Part model, mm, in its own coordinate system. A direction names the side the tool comes from. Coordinates: 2 decimals unless noted, no trailing zeros. Write each loop counter-clockwise with the first axis right and the second up, starting at its lowest first coordinate (ties: lowest second). Pieces come first, ordered by that corner, then holes. Notation, with made-up numbers: (8.5, 84.25) -> (57.5, 84.25) arc R18 cw to (57.5, 113.25) -> close; hole circle Ø8 at (89, -5). An arc over 180 degrees is marked (long way). Write item = value, one per line.
from build123d import *

# Parameters (mm, degrees)
SALIENTE_EXTRUIR1_DEPTH = 2
CORTAR_EXTRUIR1_START   = -2
CORTAR_EXTRUIR1_DEPTH   = 2


with BuildPart() as part:
    # Croquis1 → Saliente-Extruir1 (new body)
    with BuildSketch(Plane.XY):
        with BuildLine():
            Line((-39.554396855, 20.88242961), (-39.554396855, 1.28242961))
            ThreePointArc((-39.554396855, 1.28242961), (-38.763585164, -0.626758699), (-36.854396855, -1.41757039))
            Line((-36.854396855, -1.41757039), (-12.254396855, -1.41757039))
            ThreePointArc((-12.254396855, -1.41757039), (-10.345208546, -0.626758699), (-9.554396855, 1.28242961))
            Line((-9.554396855, 1.28242961), (-9.554396855, 20.88242961))
            ThreePointArc((-9.554396855, 20.88242961), (-10.345208546, 22.791617919), (-12.254396855, 23.58242961))
            Line((-12.254396855, 23.58242961), (-36.854396855, 23.58242961))
            ThreePointArc((-36.854396855, 23.58242961), (-38.763585164, 22.791617919), (-39.554396855, 20.88242961))
        make_face()
        with BuildLine():
            Line((-14.554396855, 18.90242961), (-34.554396855, 18.90242961))
            ThreePointArc((-34.554396855, 18.90242961), (-35.654396855, 17.80242961), (-34.554396855, 16.70242961))
            Line((-34.554396855, 16.70242961), (-14.554396855, 16.70242961))
            ThreePointArc((-14.554396855, 16.70242961), (-13.454396855, 17.80242961), (-14.554396855, 18.90242961))
        make_face(mode=Mode.SUBTRACT)
        with BuildLine():
            Line((-34.554396855, 3.26242961), (-14.554396855, 3.26242961))
            ThreePointArc((-14.554396855, 3.26242961), (-13.454396855, 4.36242961), (-14.554396855, 5.46242961))
            Line((-14.554396855, 5.46242961), (-34.554396855, 5.46242961))
            ThreePointArc((-34.554396855, 5.46242961), (-35.654396855, 4.36242961), (-34.554396855, 3.26242961))
        make_face(mode=Mode.SUBTRACT)
    extrude(amount=SALIENTE_EXTRUIR1_DEPTH)

    # Croquis2 → Cortar-Extruir1 (cut)
    with BuildSketch(Plane.XY.offset(2).offset(CORTAR_EXTRUIR1_START)):
        with BuildLine():
            Line((-39.554396855, 20.88242961), (-39.554396855, 1.28242961))
            ThreePointArc((-39.554396855, 1.28242961), (-38.763585164, -0.626758699), (-36.854396855, -1.41757039))
            Line((-36.854396855, -1.41757039), (-12.254396855, -1.41757039))
            ThreePointArc((-12.254396855, -1.41757039), (-10.345208546, -0.626758699), (-9.554396855, 1.28242961))
            Line((-9.554396855, 1.28242961), (-9.554396855, 20.88242961))
            ThreePointArc((-9.554396855, 20.88242961), (-10.345208546, 22.791617919), (-12.254396855, 23.58242961))
            Line((-12.254396855, 23.58242961), (-36.854396855, 23.58242961))
            ThreePointArc((-36.854396855, 23.58242961), (-38.763585164, 22.791617919), (-39.554396855, 20.88242961))
        make_face()
        with BuildLine():
            Line((-39.204396855, 20.88242961), (-39.204396855, 1.28242961))
            ThreePointArc((-39.204396855, 1.28242961), (-38.516097791, -0.379271326), (-36.854396855, -1.06757039))
            Line((-36.854396855, -1.06757039), (-12.254396855, -1.06757039))
            ThreePointArc((-12.254396855, -1.06757039), (-10.592695919, -0.379271326), (-9.904396855, 1.28242961))
            Line((-9.904396855, 1.28242961), (-9.904396855, 20.88242961))
            ThreePointArc((-9.904396855, 20.88242961), (-10.592695919, 22.544130546), (-12.254396855, 23.23242961))
            Line((-12.254396855, 23.23242961), (-36.854396855, 23.23242961))
            ThreePointArc((-36.854396855, 23.23242961), (-38.516097791, 22.544130546), (-39.204396855, 20.88242961))
        make_face(mode=Mode.SUBTRACT)
    extrude(amount=CORTAR_EXTRUIR1_DEPTH, mode=Mode.SUBTRACT)


solid = part.part
Q1. Saw through at C-C on y = 18.5. Give the cut face in (x, z), and give its area (3 significant figures).
Model answer:
outline = (-39.2, 0) -> (-35.4, 0) -> (-35.4, 2) -> (-39.2, 2) -> close; (-13.7, 0) -> (-9.9, 0) -> (-9.9, 2) -> (-13.7, 2) -> close
area = 15.2 mm²
Q2. Which spindle directions (+Z, -Z, +X, -X, +Y, -Y) get a long thin tool onto all of the face, cutting with end or side? Do faces 4 (the face through (-10.575, 22.526, 0.986)), 5 (the face through (-25, 3.262, 1)). Say none if no direction does.
Model answer:
face_4 = +Z, -Z, +X, +Y
face_5 = +Z, -Z
Q3. Mould opens along X. For faces 1 (the face through (-25, -1.068, 1)), 2 (the face through (-39.204, 11, 1)), 3 (the face through (-13.455, 4.338, 0.986)) say: released by +X, released by -X, zero draft, split by the parting line, or undercut.
Model answer:
face_1 = zero draft
face_2 = released by -X
face_3 = undercut
Q4. Probe line 1 (Y direction, x = -25.75, z = 0.2); line 2 (Y direction, x = -14, z = 1); line 3 (X direction, y = 18.25, z = 0.25). List the from-to ranges inside material, lowest first. Write a range as from..to.
Model answer:
line_1 = -1.07..3.26, 5.46..16.7, 18.9..23.23
line_2 = -1.07..3.41, 5.31..16.85, 18.75..23.23
line_3 = -39.2..-35.56, -13.55..-9.9
Q5. Saw through at D-D on y = 4.75. Give the cut face in (x, z), and give its area (3 significant figures).
Model answer:
outline = (-39.2, 0) -> (-35.58, 0) -> (-35.58, 2) -> (-39.2, 2) -> close; (-13.52, 0) -> (-9.9, 0) -> (-9.9, 2) -> (-13.52, 2) -> close
area = 14.5 mm²
Q6. Saw through at B-B on z = 0.7. Give the cut face in (x, y).
Model answer:
outline = (-39.2, 1.28) arc R2.35 ccw to (-36.85, -1.07) -> (-12.25, -1.07) arc R2.35 ccw to (-9.9, 1.28) -> (-9.9, 20.88) arc R2.35 ccw to (-12.25, 23.23) -> (-36.85, 23.23) arc R2.35 ccw to (-39.2, 20.88) -> close; hole (-34.55, 3.26) -> (-14.55, 3.26) arc R1.1 ccw to (-14.55, 5.46) -> (-34.55, 5.46) arc R1.1 ccw to start; hole (-34.55, 16.7) -> (-14.55, 16.7) arc R1.1 ccw to (-14.55, 18.9) -> (-34.55, 18.9) arc R1.1 ccw to start
Q7. Saw through at A-A on x = -16. Give the cut face in (y, z), and give its area (3 significant figures).
Model answer:
outline = (-1.07, 0) -> (3.26, 0) -> (3.26, 2) -> (-1.07, 2) -> close; (5.46, 0) -> (16.7, 0) -> (16.7, 2) -> (5.46, 2) -> close; (18.9, 0) -> (23.23, 0) -> (23.23, 2) -> (18.9, 2) -> close
area = 39.8 mm²
